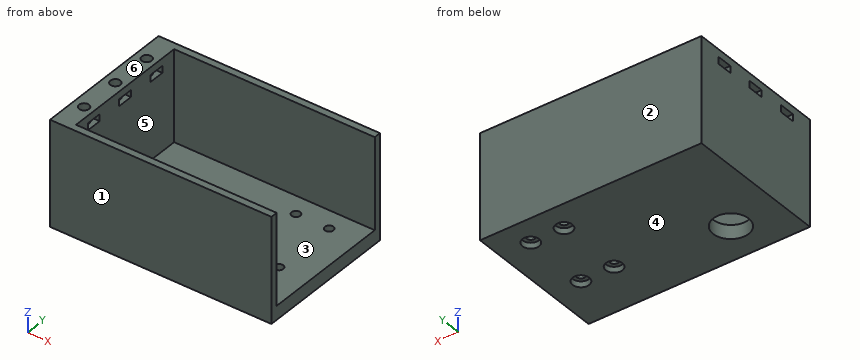
```python
from build123d import *

# Parameters (mm, degrees)
ESQUISSE3_W                                        = 80
ESQUISSE3_H                                        = 52
BOSS_EXTRU_1_DEPTH                                 = 5
ESQUISSE4_R                                        = 6.4
ENL_V_MAT_EXTRU_1_DEPTH                            = 10
BOSS_EXTRU_2_DEPTH                                 = 33
CHAMBRAGE_POUR_VIS_T_TE_RONDE_BOMB_E_M_D           = 3.1
CHAMBRAGE_POUR_VIS_T_TE_RONDE_BOMB_E_M_CBORE_D     = 6
CHAMBRAGE_POUR_VIS_T_TE_RONDE_BOMB_E_M_CBORE_DEPTH = 2.1
R_P_TITION_LIN_AIRE1_COUNT                         = 2
R_P_TITION_LIN_AIRE1_PITCH                         = 12
R_P_TITION_LIN_AIRE1_COUNT_DIR2                    = 2
R_P_TITION_LIN_AIRE1_PITCH_DIR2                    = 24
ENL_V_MAT_EXTRU_2_REACH                            = 94.304
ESQUISSE11_W                                       = 2.5
ESQUISSE11_H                                       = 5.7
R_P_TITION_LIN_AIRE2_COUNT                         = 3
R_P_TITION_LIN_AIRE2_PITCH                         = 15
R_P_TITION_LIN_AIRE3_COUNT                         = 3
R_P_TITION_LIN_AIRE3_PITCH                         = 15


with BuildPart() as part:
    # Esquisse3 → Boss.-Extru.1 (new body)
    with BuildSketch(Plane.XY):
        Rectangle(ESQUISSE3_W, ESQUISSE3_H)
    extrude(amount=BOSS_EXTRU_1_DEPTH)

    # Esquisse4 → Enlèv. mat.-Extru.1 (cut)
    with BuildSketch(Plane.XY.offset(5)):
        with Locations((-22, -12)):
            Circle(ESQUISSE4_R)
    extrude(amount=-ENL_V_MAT_EXTRU_1_DEPTH, mode=Mode.SUBTRACT)

    # Esquisse5 → Boss.-Extru.2 (add)
    with BuildSketch(Plane.XY.offset(5)):
        Polygon((-40, -26), (40, -26), (40, -23.5), (-32.5, -23.5), (-32.5, 23.5), (40, 23.5), (40, 26), (-40, 26), align=None)
    extrude(amount=BOSS_EXTRU_2_DEPTH)

    # Chambrage pour vis à tête ronde bombée M2.51 (through all)
    with Locations(Plane(origin=(0, 0, 0), x_dir=(-1, 0, 0), z_dir=(0, 0, -1))):
        with Locations((-17, 16.25)):
            chambrage_pour_vis_t_te_ronde_bomb_e_m = CounterBoreHole(CHAMBRAGE_POUR_VIS_T_TE_RONDE_BOMB_E_M_D / 2, CHAMBRAGE_POUR_VIS_T_TE_RONDE_BOMB_E_M_CBORE_D / 2, CHAMBRAGE_POUR_VIS_T_TE_RONDE_BOMB_E_M_CBORE_DEPTH)

    # Répétition linéaire1: Chambrage pour vis _ t_te ronde bomb_e M 2 × 2
    with Locations(*[(i * R_P_TITION_LIN_AIRE1_PITCH, -j * R_P_TITION_LIN_AIRE1_PITCH_DIR2, 0) for i in range(R_P_TITION_LIN_AIRE1_COUNT) for j in range(R_P_TITION_LIN_AIRE1_COUNT_DIR2) if (i, j) != (0, 0)]):
        add(chambrage_pour_vis_t_te_ronde_bomb_e_m, mode=Mode.SUBTRACT)

    # Esquisse11 → Enlèv. mat.-Extru.2 (cut, up to next)
    with BuildSketch(Plane.ZY.offset(40), mode=Mode.PRIVATE) as enl_v_mat_extru_2_sk1:
        with Locations((34.05, 15)):
            Rectangle(ESQUISSE11_W, ESQUISSE11_H)
    enl_v_mat_extru_2_tool1 = extrude(enl_v_mat_extru_2_sk1.sketch, amount=-ENL_V_MAT_EXTRU_2_REACH, mode=Mode.PRIVATE) & part.part
    enl_v_mat_extru_2 = enl_v_mat_extru_2_tool1.solids().sort_by_distance((-40, 15, 34.05))[0]
    add(enl_v_mat_extru_2, mode=Mode.SUBTRACT)

    # Répétition linéaire2: Enlèv. mat.-Extru.2 ×3
    with Locations(*[(0, -i * R_P_TITION_LIN_AIRE2_PITCH, 0) for i in range(1, R_P_TITION_LIN_AIRE2_COUNT)]):
        add(enl_v_mat_extru_2, mode=Mode.SUBTRACT)

    # Esquisse15 → Dégagement M31 (revolve, cut)
    with BuildSketch(Plane(origin=(-36, 15, 38), x_dir=(0, -1, 0), z_dir=(1, 0, 0))):
        Polygon((0, 0), (0, 7.431549114), (1.8, 6.35), (1.8, 0), align=None)
    d_gagement_m31 = revolve(axis=Axis((-36, 15, 44.35), (0, 0, -1)), mode=Mode.SUBTRACT)

    # Répétition linéaire3: Dégagement M31 ×3
    with Locations(*[(0, -i * R_P_TITION_LIN_AIRE3_PITCH, 0) for i in range(1, R_P_TITION_LIN_AIRE3_COUNT)]):
        add(d_gagement_m31, mode=Mode.SUBTRACT)


solid = part.part
```
Part model, mm, in its own coordinate system. Face numbers are marked on the shaded views. A direction names the side the tool comes from. Round coordinates to 2 decimals unless told otherwise and drop trailing zeros. Order: outer loops, then holes, each group sorted by start corner. A loop starts at its lowest first (then second) coordinate and runs counter-clockwise, first axis right, second up. Notation, with made-up numbers: M 38,12 L 55,12 A17 ccw 55,31 Z; hole C 78,-32.5 d10. An arc over 180 degrees is marked long. Put each result on its own line as item: value. Start each with the question number.
1. Drop flat-ended pins along their axis: pin 1 (4 mm diameter, centred on y = 15.5, z = 21.5, fed in from +X); pin 2 (5 mm diameter, centred on x = 29.5, y = -8.5, fed in from -Z); pin 3 (14 mm diameter, centred on x = 11.5, y = 7.5, fed in from +Z); pin 4 (5 mm diameter, centred on x = 17, y = 16.25, fed in from -Z). Give the stop position or say it passes through.
2. Slice it at D-D on y = 9.5. List the corners of the cut face in (x, z), then the cut area to 4 significant figures.
3. Two-plate mould, pull along Y, no slides. Class the marked faces 1, 2, 3 and 4: +Y half, -Y half, draft (parallel to the pull), parting line (faces both ways), or undercut.
4. Slice it at B-B on z = 25. List the corners of the cut face in (x, y).
5. Slice it at A-A on x = 17. List the corners of the cut face in (y, z), then the cut area to 3 significant figures.
6. Tool access for the marked faces 5 and 6: list every direction of +Z, -Z, +X, -X, +Y, -Y with a clear straight run to the whole face (end or side of a thin tool).
7. Slice it at C-C on x = 2. List the corners of the cut face in (y, z).
8. Drill centre lines: probe 1 along X at (y, z) = (16, 4); probe 2 along Y at (x, z) = (29, 3.1); probe 3 along Y at (x, z) = (29, 1.5). Where is each one in solid material? Low to high. Write a range as [from, to].
Findings:
1. pin 1: x = -32.5
1. pin 2: z = 0
1. pin 3: z = 5
1. pin 4: z = 2.1
2. outline: M -40,0 L 40,0 L 40,5 L -32.5,5 L -32.5,38 L -40,38 Z
2. area: 647.5 mm2
3. face 1: -Y half
3. face 2: +Y half
3. face 3: undercut
3. face 4: draft
4. outline: M -40,-26 L 40,-26 L 40,-23.5 L -32.5,-23.5 L -32.5,23.5 L 40,23.5 L 40,26 L -40,26 Z
5. outline: M -26,0 L -10.75,0 L -10.75,2.1 L -9.3,2.1 L -9.3,5 L -23.5,5 L -23.5,38 L -26,38 Z; M -6.2,2.1 L -4.75,2.1 L -4.75,0 L 13.25,0 L 13.25,2.1 L 14.7,2.1 L 14.7,5 L -6.2,5 Z; M 17.8,2.1 L 19.25,2.1 L 19.25,0 L 26,0 L 26,38 L 23.5,38 L 23.5,5 L 17.8,5 Z
5. area: 382 mm2
6. face 5: +Z, +X
6. face 6: +Z, +X, -X, +Y, -Y
7. outline: M -26,0 L 26,0 L 26,38 L 23.5,38 L 23.5,5 L -23.5,5 L -23.5,38 L -26,38 Z
8. probe 1: [-40, 15.47], [18.53, 27.47], [30.53, 40]
8. probe 2: [-26, -9.3], [-6.2, 14.7], [17.8, 26]
8. probe 3: [-26, -10.75], [-4.75, 13.25], [19.25, 26]
